```python
from build123d import *

# Parameters (mm, degrees)
SKETCH_1_W          = 92
SKETCH_1_H          = 92
SKETCH_1_R          = 40
EXTRUDE_1_DEPTH     = 13
SKETCH_3_OUTSIDE_W  = 120.152
SKETCH_3_OUTSIDE_H  = 120.152
SKETCH_3_OUTSIDE_R  = 58
CUT_EXTRUDE_2_DEPTH = 13
SKETCH_5_R          = 4.5
CUT_EXTRUDE_3_DEPTH = 13
SKETCH_5_3_R        = 7
SKETCH_5_3_R_2      = 4.5
CUT_EXTRUDE_4_DEPTH = 8.1
CHAMFER_1_SIZE      = 0.4
SKETCH_7_R          = 40
SKETCH_7_R_2        = 38.6
EXTRUDE_2_DEPTH     = 100
FILLET_1_R          = 0.8
CHAMFER_2_SIZE      = 0.3
FILLET_2_R          = 0.4


with BuildPart() as part:
    # Sketch 1 → Extrude 1 (new body)
    with BuildSketch(Plane.XY):
        Rectangle(SKETCH_1_W, SKETCH_1_H)
        Circle(SKETCH_1_R, mode=Mode.SUBTRACT)
    extrude(amount=EXTRUDE_1_DEPTH)

    # Sketch 3 outside → Cut-Extrude 2 (cut)
    with BuildSketch(Plane.XY.offset(13)):
        Rectangle(SKETCH_3_OUTSIDE_W, SKETCH_3_OUTSIDE_H)
        Circle(SKETCH_3_OUTSIDE_R, mode=Mode.SUBTRACT)
    extrude(amount=-CUT_EXTRUDE_2_DEPTH, mode=Mode.SUBTRACT)

    # Sketch 5 → Cut-Extrude 3 (cut)
    with BuildSketch(Plane.XY):
        with Locations(Location((-34.648232278, 34.648232278, 0), (0, 0, 180))):  # turned: the seam where the file's is
            Circle(SKETCH_5_R)
        with Locations(Location((-34.648232278, -34.648232278, 0), (0, 0, 180))):  # turned: the seam where the file's is
            Circle(SKETCH_5_R)
        with Locations(Location((34.648232278, -34.648232278, 0), (0, 0, 180))):  # turned: the seam where the file's is
            Circle(SKETCH_5_R)
        with Locations(Location((34.648232278, 34.648232278, 0), (0, 0, 180))):  # turned: the seam where the file's is
            Circle(SKETCH_5_R)
    extrude(amount=CUT_EXTRUDE_3_DEPTH, mode=Mode.SUBTRACT)

    # Sketch 5_3 → Cut-Extrude 4 (cut)
    with BuildSketch(Plane.XY):
        with Locations((-34.648232278, 34.648232278)):
            Circle(SKETCH_5_3_R)
        with Locations(Location((-34.648232278, 34.648232278, 0), (0, 0, 180))):  # turned: the seam where the file's is
            Circle(SKETCH_5_3_R_2, mode=Mode.SUBTRACT)
        with Locations(Location((34.648232278, 34.648232278, 0), (0, 0, 180))):  # turned: the seam where the file's is
            Circle(SKETCH_5_3_R)
        with Locations(Location((34.648232278, 34.648232278, 0), (0, 0, 180))):  # turned: the seam where the file's is
            Circle(SKETCH_5_3_R_2, mode=Mode.SUBTRACT)
        with Locations((34.648232278, -34.648232278)):
            Circle(SKETCH_5_3_R)
        with Locations(Location((34.648232278, -34.648232278, 0), (0, 0, 180))):  # turned: the seam where the file's is
            Circle(SKETCH_5_3_R_2, mode=Mode.SUBTRACT)
        with Locations(Location((-34.648232278, -34.648232278, 0), (0, 0, 180))):  # turned: the seam where the file's is
            Circle(SKETCH_5_3_R)
        with Locations(Location((-34.648232278, -34.648232278, 0), (0, 0, 180))):  # turned: the seam where the file's is
            Circle(SKETCH_5_3_R_2, mode=Mode.SUBTRACT)
    extrude(amount=CUT_EXTRUDE_4_DEPTH, mode=Mode.SUBTRACT)

    # Chamfer 1
    chamfer_1_edges = [part.edges().sort_by_distance(p)[0] for p in [
        (41.648232278, 34.648232278, 0),
        (-41.648232278, 34.648232278, 0),
        (-40, 0, 0),
        (-40, 0, 13),
        (0, -46, 0),
        (0, -46, 13),
        (-46, 0, 0),
        (-46, 0, 13),
        (0, 46, 0),
        (0, 46, 13),
        (46, 0, 0),
        (46, 0, 13),
        (41.012193309, -41.012193309, 13),
        (41.012193309, 41.012193309, 13),
        (-41.012193309, 41.012193309, 13),
        (-41.012193309, -41.012193309, 13),
        (41.012193309, 41.012193309, 0),
        (-41.012193309, 41.012193309, 0),
        (41.012193309, -41.012193309, 0),
        (-41.012193309, -41.012193309, 0),
        (39.148232278, 34.648232278, 13),
        (39.148232278, -34.648232278, 13),
        (-30.148232278, -34.648232278, 13),
        (-30.148232278, 34.648232278, 13),
        (-27.648232278, -34.648232278, 0),
        (27.648232278, -34.648232278, 0),
    ]]
    chamfer(chamfer_1_edges, length=CHAMFER_1_SIZE)

    # Sketch 7 → Extrude 2 (add)
    with BuildSketch(Plane(origin=(0, 0, 0), x_dir=(-1, 0, 0), z_dir=(0, 0, -1))):
        Circle(SKETCH_7_R)
        Circle(SKETCH_7_R_2, mode=Mode.SUBTRACT)
    extrude(amount=-EXTRUDE_2_DEPTH)

    # Fillet 1
    fillet_1_edges = [part.edges().sort_by_distance(p)[0] for p in [
        (40, 0, 100),
    ]]
    fillet(fillet_1_edges, radius=FILLET_1_R)

    # Chamfer 2
    chamfer_2_edges = [part.edges().sort_by_distance(p)[0] for p in [
        (38.6, 0, 100),
    ]]
    chamfer(chamfer_2_edges, length=CHAMFER_2_SIZE)

    # Sketch 8 → Revolve 1 (revolve)
    with BuildSketch(Plane(origin=(0, 0, 0), x_dir=(0, 0, -1), z_dir=(1, 0, 0)), mode=Mode.PRIVATE) as revolve_1_sk:
        Polygon((-97.3, 38.6), (-2.4, 38.6), (-2.4, 37.4), (-1.2, 37.4), (-1.2, 26.5), (0, 26.5), (0, 25), (-99.7, 25), (-99.7, 26.5), (-98.5, 26.5), (-98.5, 37.4), (-97.3, 37.4), align=None)
    revolve(revolve_1_sk.sketch.rotate(Axis((0, 0, 0), (0, 0, 1)), 90), axis=Axis((0, 0, 0), (0, 0, 1)))  # turned: the seam where the file's is

    # Fillet 2
    fillet_2_edges = [part.edges().sort_by_distance(p)[0] for p in [
        (-35.327043465, 46, 6.5),
        (-46, 35.327043465, 6.5),
        (-46, -35.327043465, 6.5),
        (-35.327043465, -46, 6.5),
        (35.327043465, -46, 6.5),
        (46, -35.327043465, 6.5),
        (46, 35.327043465, 6.5),
        (35.327043465, 46, 6.5),
    ]]
    fillet(fillet_2_edges, radius=FILLET_2_R)


solid = part.part
```
Geometry check sheet. Reference: the model listing, model coordinates, mm. A direction names the side the tool comes from. Round coordinates to 2 decimals unless told otherwise and drop trailing zeros. Loops run counter-clockwise (first coordinate to the right, second up) from the corner with the lowest first, then second, coordinate; pieces in that order, holes last. Notation, with made-up numbers: (3.5, 19.25) -> (32.5, 19.25) arc R28 cw to (32.5, 49.25) -> close; hole circle Ø3 at (81, 51.25). An arc over 180 degrees is marked (long way). Use a Markdown table: item, result.
(1) Set-up check for faces 1 (the cylindrical face through (-36.82, 11.59, 1.18)), 2 (the conical face through (-40.884, -40.735, 12.886)), 3 (the flat face through (20, -16, 99.7)): record each of +Z, -Z, +X, -X, +Y, -Y from which the full face is reachable in a straight line by a thin tool's end or side.
Calculated:
| item | result |
|---|---|
| face 1 | -Z |
| face 2 | +Z, -X, -Y |
| face 3 | +Z |
(2) Scan lines: probe 1 along X at (y, z) = (-22, 55); probe 2 along Y at (x, z) = (17.5, 45); probe 3 along Z at (x, y) = (16, 40.5). Record each from-to range of solid material in increasing order.
Calculated:
| item | result |
|---|---|
| probe 1 | -33.41 to -11.87, 11.87 to 33.41 |
| probe 2 | -35.97 to -17.85, 17.85 to 35.97 |
| probe 3 | 0 to 13 |
(3) Go/stop test with flat-tipped pins: P1, Ø6, axis at x = 5, y = -20.5, coming from the -Z side; P2, Ø3, axis at x = -26.5, z = 75, coming from the -Y side (3 decimals); P3, Ø7, axis at x = -36.5, y = 31, coming from the -Z side; P4, Ø11.5, axis at x = 34.65, y = 34.65, coming from the +Z side. Record where each tip stops, or that it passes through.
Calculated:
| item | result |
|---|---|
| P1 | through |
| P2 | y = -31.225 |
| P3 | z = 0 |
| P4 | z = 13 |
(4) Sectioned sample at A-A (z = 27). Enter the section's corners in (x, y).
Calculated:
| item | result |
|---|---|
| outline | circle Ø80 at (0, 0); hole circle Ø50 at (0, 0) |
(5) Sectioned sample at B-B (x = -32.5). Give the number of separate pieces and of enclosed holes in the cut face, then the cut area to 3 significant figures.
Calculated:
| item | result |
|---|---|
| separate pieces | 3 |
| enclosed holes | 0 |
| area | 4,830 mm² |
